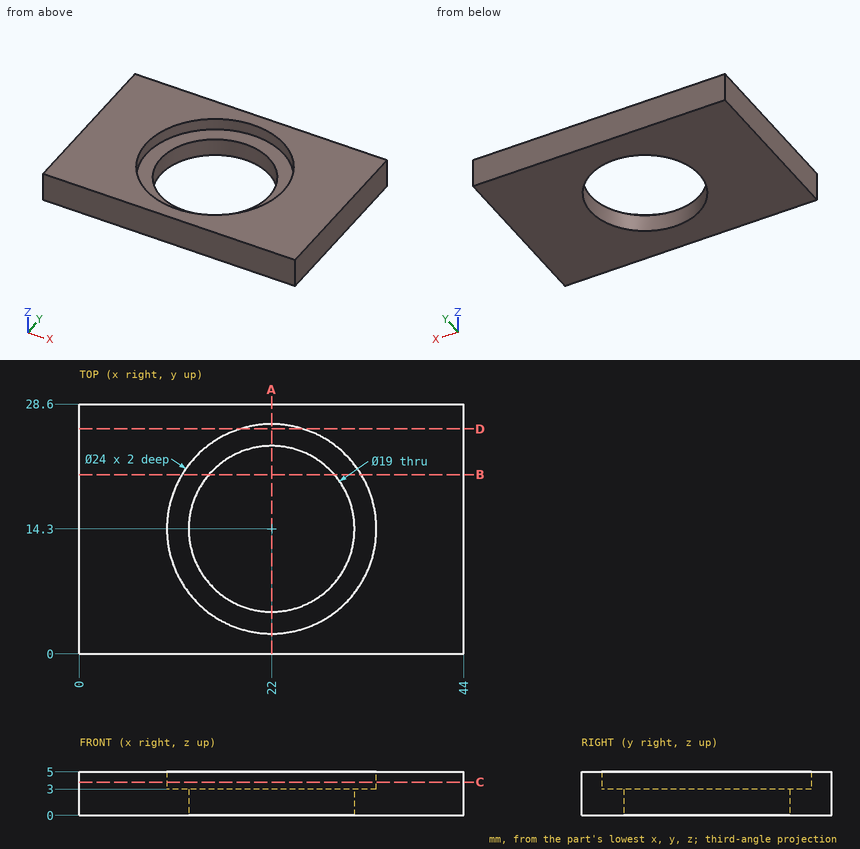
Drawing for the job (mm, zero at the part's lowest x, y, z). Coordinates: 2 decimals unless noted, no trailing zeros. Order: outer loops, then holes, each group sorted by start corner. A loop starts at its lowest first (then second) coordinate and runs counter-clockwise, first axis right, second up. Notation, with made-up numbers: (45, 71) - (101, 71) arc R16 ccw to (101, 77) - close; hole circle Ø3 at (76, -4.75). An arc over 180 degrees is marked (long way). Use a Markdown table: item, result. Add a question column.
(1) Flat gauge pins, fed straight in: pin 1 (12 mm diameter, centred on x = 32, y = 22, fed in from -Z); pin 2 (14.5 mm diameter, centred on x = 22, y = 14.3, fed in from +Z). Where does each tip first touch, or does it go through?
(2) Saw through at D-D (y = 25.75). Give the cut face in (x, z), then the cut area to 3 significant figures.
(3) Saw through at A-A (x = 22). Give the cut face in (y, z), then the cut area to 3 significant figures.
(4) Saw through at C-C (z = 3.8). Give the cut face in (x, y).
(5) Drill centre lines: line 1 along Y through (x, z) = (22, 1); line 2 along Y through (x, z) = (22, 3.7); line 3 along X through (y, z) = (14.25, 3.05). Where is each one in solid material? Low to high. Write a range as [from, to].
(6) Saw through at B-B (y = 20.5). Give the cut face in (x, z).
Solved:
| question | item | result |
|---|---|---|
| 1 | pin 1 | stops at z = 0 |
| 1 | pin 2 | passes through |
| 2 | outline | (0, 0) - (44, 0) - (44, 5) - (25.59, 5) - (25.59, 3) - (18.41, 3) - (18.41, 5) - (0, 5) - close |
| 2 | area | 206 mm² |
| 3 | outline | (0, 0) - (4.8, 0) - (4.8, 3) - (2.3, 3) - (2.3, 5) - (0, 5) - close; (23.8, 0) - (28.6, 0) - (28.6, 5) - (26.3, 5) - (26.3, 3) - (23.8, 3) - close |
| 3 | area | 38.0 mm² |
| 4 | outline | (0, 0) - (44, 0) - (44, 28.6) - (0, 28.6) - close; hole circle Ø24 at (22, 14.3) |
| 5 | line 1 | y = [0, 4.8], [23.8, 28.6] |
| 5 | line 2 | y = [0, 2.3], [26.3, 28.6] |
| 5 | line 3 | x = [0, 10], [34, 44] |
| 6 | outline | (0, 0) - (14.8, 0) - (14.8, 3) - (11.73, 3) - (11.73, 5) - (0, 5) - close; (29.2, 0) - (44, 0) - (44, 5) - (32.27, 5) - (32.27, 3) - (29.2, 3) - close |
